from build123d import *

# Parameters (mm, degrees)
F0_R          = 15.5
F1_DEPTH      = 114.3
F1_DEPTH_BACK = 114.3
F2_R          = 17.6785322686
F2_R_2        = 15.5
F3_DEPTH      = 25
F4_R          = 5


# Not quite as in the source:
# - a pattern or mirror of a feature is missing from the dataset's text; its kind, count and spacing are read off the source's solid


with BuildPart() as f1:
    # F0 (on Top) → F1 (new body, two sides)
    with BuildSketch(Plane.XY) as f1_sk:
        Circle(F0_R)
    extrude(amount=F1_DEPTH)
    extrude(f1_sk.sketch, amount=-F1_DEPTH_BACK)

    # F2 (on face) → F3 (join)
    with BuildSketch(Plane.XY.offset(114.3)):
        Circle(F2_R)
        Circle(F2_R_2, mode=Mode.SUBTRACT)
        Circle(F2_R_2)
    f3 = extrude(amount=-F3_DEPTH)

    # F3_copies: F3 across plane
    add(f3.mirror(Plane(origin=(0, 0, 0), x_dir=(-1, 0, 0), z_dir=(0, 0, -1))))

    # F4
    f4_edges = [f1.edges().sort_by_distance(p)[0] for p in [
        (-17.678532, 0, 114.3),
        (-17.678532, 0, -114.3),
    ]]
    fillet(f4_edges, radius=F4_R)


solid = f1.part
Can you work these out from the model? Positions are in its coordinate system, mm. A direction names the side the tool comes from. Round coordinates to 2 decimals unless told otherwise and drop trailing zeros. Loops run counter-clockwise (first coordinate to the right, second up) from the corner with the lowest first, then second, coordinate; pieces in that order, holes last. Notation, with made-up numbers: (38, 54.25) - (86, 54.25) arc R34 ccw to (86, 86.25) - close; hole circle Ø2 at (-18, 64). An arc over 180 degrees is marked (long way). Answer in a Markdown table with one row per item. Add a question column.
Q1. We'd pull the mould along Z, two halves only. Please class faces 3 (the flat face through (0, 0, 114.3)), 4 (the flat face through (0, -16, 89.3)), 5 (the cylindrical face through (-2.018, 15.368, 1.25)), 6 (the cylindrical face through (16.862, 5.31, 99.44)): pulls with the +Z half, pulls with the -Z half, needs draft (parallel to the pull), parting line crosses it, or undercut.
Q2. For pin 1 Ø2 at (x, z) = (5, 23.5) entering from +Y (3 decimals); pin 2 Ø5 at (y, z) = (8.5, 3) entering from +X; pin 3 Ø5 at (x, z) = (1, -19) entering from -Y, each with a flat end and sliding along its axis, tell me the tip position at first contact or that it passes through.
Q3. I need wall thicknesses on L1, parallel to X at y = 1, z = -42.5; L2, parallel to Z at x = 9, y = -14.5. Which ranges of each line are inside material? Lowest first, please.
Q4. Which directions (+Z, -Z, +X, -X, +Y, -Y) give clear straight access to the entire face, cutting with the end or side of a thin tool? Please do faces 1 (the cylindrical face through (16.862, 5.31, -99.44)), 2 (the flat face through (0, -16, -89.3)).
Q5. I want a section at A-A on x = 0. List the corners of the cut face in (y, z) for me.
Q6. I want a section at C-C on z = 84. List the corners of the cut face in (x, y) for me, and give its area (3 significant figures).
A:
| question | item | result |
|---|---|---|
| 1 | face 3 | pulls with the +Z half |
| 1 | face 4 | undercut |
| 1 | face 5 | undercut |
| 1 | face 6 | needs draft |
| 2 | pin 1 | y = 14.975 |
| 2 | pin 2 | x = 14.29 |
| 2 | pin 3 | y = -15.5 |
| 3 | L1 | -15.47 to 15.47 |
| 3 | L2 | -111.7 to -89.3, 89.3 to 111.7 |
| 4 | face 1 | +Z, -Z |
| 4 | face 2 | none |
| 5 | outline | (-17.68, -109.3) arc R5 ccw to (-12.68, -114.3) - (12.68, -114.3) arc R5 ccw to (17.68, -109.3) - (17.68, -89.3) - (15.5, -89.3) - (15.5, 89.3) - (17.68, 89.3) - (17.68, 109.3) arc R5 ccw to (12.68, 114.3) - (-12.68, 114.3) arc R5 ccw to (-17.68, 109.3) - (-17.68, 89.3) - (-15.5, 89.3) - (-15.5, -89.3) - (-17.68, -89.3) - close |
| 6 | outline | circle Ø31 at (0, 0) |
| 6 | area | 755 mm^2 |
